Study the drawing (mm; zero at the part's minimum x, y, z) and answer. A direction names the side the tool comes from. Round coordinates to 2 decimals unless told otherwise and drop trailing zeros. Write each loop counter-clockwise with the first axis right and the second up, starting at its lowest first coordinate (ties: lowest second). Pieces come first, ordered by that corner, then holes. Notation, with made-up numbers: (-20.5, -33.5) -> (2.5, -33.5) arc R21 cw to (2.5, -1.5) -> close; hole circle Ø9 at (63, -5). An arc over 180 degrees is marked (long way). Write each question's results on one line, items separated by ' | '. Start each with the question number.
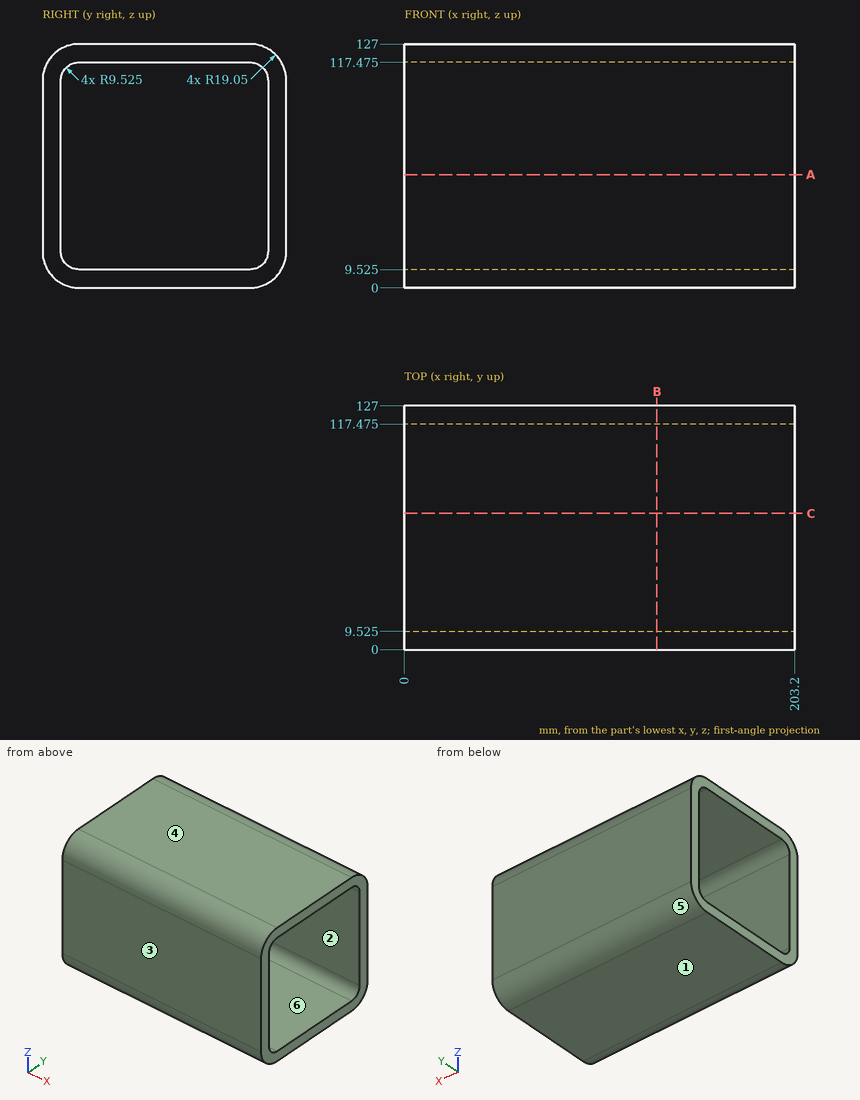
Q1. The part is cut by section A-A, the plane z = 59. Write down the section's boundary in (x, y) (3 decimals), then the cut area to 3 significant figures.
Q2. Determine the mould class of the marked faces 3, 4, 5 and 6 for opening direction Y: pulls with the +Y half, pulls with the -Y half, needs draft (parallel to the pull), parting line crosses it, or undercut.
Q3. Find the intervals of material crossed by line 1 (Z direction, x = 84.5, y = 62) (3 decimals); line 2 (Y direction, x = 48, z = 114), in increasing order.
Q4. For the marked faces 1 and 2, determine the directions among +Z, -Z, +X, -X, +Y, -Y from which every point of the face is accessible in a straight line to the end or side of a thin tool.
Q5. The part is cut by section B-B, the plane x = 131.5. Write down the section's boundary in (y, z) (3 decimals).
Answers follow:
1) outline: (0, 0) -> (203.2, 0) -> (203.2, 9.525) -> (0, 9.525) -> close; (0, 117.475) -> (203.2, 117.475) -> (203.2, 127) -> (0, 127) -> close | area: 3,870 mm^2
2) face 3: pulls with the -Y half | face 4: needs draft | face 5: pulls with the +Y half | face 6: undercut
3) line 1: 0 to 9.525, 117.475 to 127 | line 2: 0.99 to 11.69, 115.31 to 126.01
4) face 1: -Z, +X, -X, +Y, -Y | face 2: +X, -X
5) outline: (0, 19.05) arc R19.05 ccw to (19.05, 0) -> (107.95, 0) arc R19.05 ccw to (127, 19.05) -> (127, 107.95) arc R19.05 ccw to (107.95, 127) -> (19.05, 127) arc R19.05 ccw to (0, 107.95) -> close; hole (9.525, 19.05) arc R9.525 ccw to (19.05, 9.525) -> (107.95, 9.525) arc R9.525 ccw to (117.475, 19.05) -> (117.475, 107.95) arc R9.525 ccw to (107.95, 117.475) -> (19.05, 117.475) arc R9.525 ccw to (9.525, 107.95) -> close
